Check sheet for the modelled part. Datum: model origin and axes. Units: mm. A direction names the side the tool comes from. Give positions to 0.01 mm unless a question says otherwise; leave off trailing zeros. Write each loop counter-clockwise with the first axis right and the second up, starting at its lowest first coordinate (ties: lowest second). Pieces come first, ordered by that corner, then holes. Notation, with made-up numbers: (58.25, -19) -> (87.25, -19) arc R20 ccw to (87.25, 20) -> close; hole circle Ø2 at (89.25, -28). An arc over 180 degrees is marked (long way). Return JSON: item names as keys, results as strings.
from build123d import *

# Parameters (mm, degrees)
SKETCH1_R           = 10.5
BOSS_EXTRUDE1_DEPTH = 2
SKETCH2_R           = 4.5
SKETCH2_R_2         = 3
BOSS_EXTRUDE2_DEPTH = 3
SKETCH3_R           = 1
CUT_EXTRUDE1_DEPTH  = 3
SKETCH4_R           = 4.25
SKETCH4_R_2         = 3.25
SKETCH4_R_3         = 2.75
SKETCH4_R_4         = 1
CUT_EXTRUDE2_DEPTH  = 0.5
SKETCH5_R           = 0.75
CUT_EXTRUDE3_DEPTH  = 2.5
SKETCH7_R           = 0.75
CUT_EXTRUDE4_DEPTH  = 2.5


with BuildPart() as part:
    # Sketch1 → Boss-Extrude1 (new body)
    with BuildSketch(Plane(origin=(0, 0, 0), x_dir=(1, 0, 0), z_dir=(0, 1, 0))):
        Circle(SKETCH1_R)
    extrude(amount=BOSS_EXTRUDE1_DEPTH)

    # Sketch2 → Boss-Extrude2 (add)
    with BuildSketch(Plane(origin=(0, 2, 0), x_dir=(1, 0, 0), z_dir=(0, 1, 0))):
        Circle(SKETCH2_R)
        Circle(SKETCH2_R_2, mode=Mode.SUBTRACT)
    extrude(amount=BOSS_EXTRUDE2_DEPTH)

    # Sketch3 → Cut-Extrude1 (cut)
    with BuildSketch(Plane(origin=(0, 2, 0), x_dir=(1, 0, 0), z_dir=(0, 1, 0))):
        Circle(SKETCH3_R)
    extrude(amount=-CUT_EXTRUDE1_DEPTH, mode=Mode.SUBTRACT)

    # Sketch4 → Cut-Extrude2 (cut)
    with BuildSketch(Plane.XZ):
        Circle(SKETCH4_R)
        Circle(SKETCH4_R_2, mode=Mode.SUBTRACT)
        Circle(SKETCH4_R_3)
        Circle(SKETCH4_R_4, mode=Mode.SUBTRACT)
    extrude(amount=-CUT_EXTRUDE2_DEPTH, mode=Mode.SUBTRACT)

    # Sketch5 → Cut-Extrude3 (cut)
    with BuildSketch(Plane.XZ):
        with Locations((0, 7)):
            Circle(SKETCH5_R)
        with Locations((3, 7)):
            Circle(SKETCH5_R)
        with Locations((-3, 7)):
            Circle(SKETCH5_R)
    cut_extrude3 = extrude(amount=-CUT_EXTRUDE3_DEPTH, mode=Mode.SUBTRACT)

    # Mirror1: Cut-Extrude3 across plane
    add(cut_extrude3.mirror(Plane.XY), mode=Mode.SUBTRACT)

    # Sketch7 → Cut-Extrude4 (cut)
    with BuildSketch(Plane.XZ):
        with Locations((7, 0)):
            Circle(SKETCH7_R)
        with Locations((7, 3)):
            Circle(SKETCH7_R)
        with Locations((7, -3)):
            Circle(SKETCH7_R)
    cut_extrude4 = extrude(amount=-CUT_EXTRUDE4_DEPTH, mode=Mode.SUBTRACT)

    # Mirror2: Cut-Extrude4 across plane
    add(cut_extrude4.mirror(Plane(origin=(0, 0, 0), x_dir=(0, 0, 1), z_dir=(1, 0, 0))), mode=Mode.SUBTRACT)


solid = part.part
(1) Release check for a two-part mould opening along Z. For faces 1 (the cylindrical face through (10, 1, -3.2)), 2 (the flat face through (1, 5, 3)), 3 (the cylindrical face through (-3.595, 0.986, 6.544)) record: pulls with the +Z half, pulls with the -Z half, needs draft (parallel to the pull), parting line crosses it, or undercut.
Reply:
{"face 1": "parting line crosses it", "face 2": "needs draft", "face 3": "undercut"}
(2) Cross-section at D-D on x = 7.25. Enter the section's corners in (y, z), then the cut area to 3 significant figures.
Reply:
{"outline": "(0, -7.6) -> (2, -7.6) -> (2, -3.71) -> (0, -3.71) -> close; (0, -2.29) -> (2, -2.29) -> (2, -0.71) -> (0, -0.71) -> close; (0, 0.71) -> (2, 0.71) -> (2, 2.29) -> (0, 2.29) -> close; (0, 3.71) -> (2, 3.71) -> (2, 7.6) -> (0, 7.6) -> close", "area": "21.9 mm^2"}
(3) Cross-section at B-B on x = -7. Enter the section's corners in (y, z), then the cut area to 3 significant figures.
Reply:
{"outline": "(0, -7.83) -> (2, -7.83) -> (2, -3.75) -> (0, -3.75) -> close; (0, -2.25) -> (2, -2.25) -> (2, -0.75) -> (0, -0.75) -> close; (0, 0.75) -> (2, 0.75) -> (2, 2.25) -> (0, 2.25) -> close; (0, 3.75) -> (2, 3.75) -> (2, 7.83) -> (0, 7.83) -> close", "area": "22.3 mm^2"}
(4) Depth check by flat-ended pin: pin 1 Ø1.7 at (x, z) = (-3, 7) entering from +Y; pin 2 Ø3 at (x, y) = (8.5, 2) entering from +Z; pin 3 Ø2 at (y, z) = (4, -1) entering from +X. Enter the tip coordinate at first touch or a pass-through.
Reply:
{"pin 1": "y = 2", "pin 2": "z = 7.83", "pin 3": "x = 4.5"}
(5) Set-up check for faces 4 (the cylindrical face through (-0.596, 0.246, -2.685)), 5 (the cylindrical face through (6.25, 0.99, -2.97)), 6 (the flat face through (5, 2, 0)): record each of +Z, -Z, +X, -X, +Y, -Y from which the full face is reachable in a straight line by a thin tool's end or side.
Reply:
{"face 4": "-Y", "face 5": "+Y, -Y", "face 6": "+Y"}
(6) Cross-section at A-A on y = 1.05. State how many separate pieces and enclosed holes the cut face has, then the cut area to 3 significant figures.
Reply:
{"separate pieces": "1", "enclosed holes": "13", "area": "322 mm^2"}
(7) Thickness scan on L1, parallel to X at y = 1.55, z = -7; L2, parallel to X at y = 4.2, z = 0. Record the ranges inside material, lowest first.
Reply:
{"L1": "-7.83 to -3.75, -2.25 to -0.75, 0.75 to 2.25, 3.75 to 7.83", "L2": "-4.5 to -3, 3 to 4.5"}
